from build123d import *

# Parameters (mm, degrees)
MOTOR_HOLDER_DEPTH = 15
SKETCH2_R          = 2.4
LEGO_MOUNT_DEPTH   = 7.76


with BuildPart() as part:
    # Sketch1 → Motor Holder (new body)
    with BuildSketch(Plane(origin=(0, 0, 0), x_dir=(0, 0, -1), z_dir=(1, 0, 0))):
        with BuildLine():
            Line((-8.959047103, 12.31), (8.959047103, 12.31))
            ThreePointArc((8.959047103, 12.31), (15.225, 0), (8.959047103, -12.31))
            Line((8.959047103, -12.31), (-8.959047103, -12.31))
            ThreePointArc((-8.959047103, -12.31), (-15.225, 0), (-8.959047103, 12.31))
        make_face()
        with BuildLine():
            Line((-7.923037612, 9.31), (7.923037612, 9.31))
            ThreePointArc((7.923037612, 9.31), (12.225, 0), (7.923037612, -9.31))
            Line((7.923037612, -9.31), (-7.923037612, -9.31))
            ThreePointArc((-7.923037612, -9.31), (-12.225, 0), (-7.923037612, 9.31))
        make_face(mode=Mode.SUBTRACT)
    extrude(amount=MOTOR_HOLDER_DEPTH)

    # Sketch2 → Lego Mount (add)
    # profile 1 of 2: a face of its own
    with BuildSketch(Plane.ZY):
        with BuildLine():
            Line((-7.97, 19.277326297), (7.97, 19.277326297))
            ThreePointArc((7.97, 19.277326297), (11.067073538, 16.640950889), (8.959047103, 13.162651831))
            Line((8.959047103, 13.162651831), (8.959047103, 12.31))
            Line((8.959047103, 12.31), (-8.959047103, 12.31))
            Line((-8.959047103, 12.31), (-8.959047103, 13.162651831))
            ThreePointArc((-8.959047103, 13.162651831), (-11.067073538, 16.640950889), (-7.97, 19.277326297))
        make_face()
        with Locations((-7.97, 16.14)):
            Circle(SKETCH2_R, mode=Mode.SUBTRACT)
        with Locations((0, 16.14)):
            Circle(SKETCH2_R, mode=Mode.SUBTRACT)
        with Locations((7.97, 16.14)):
            Circle(SKETCH2_R, mode=Mode.SUBTRACT)
    # profile 2 of 2: a face of its own
    with BuildSketch(Plane.ZY):
        with BuildLine():
            Line((-7.97, -19.277326297), (7.97, -19.277326297))
            ThreePointArc((7.97, -19.277326297), (11.067073538, -16.640950889), (8.959047103, -13.162651831))
            Line((8.959047103, -13.162651831), (8.959047103, -12.31))
            Line((8.959047103, -12.31), (-8.959047103, -12.31))
            Line((-8.959047103, -12.31), (-8.959047103, -13.162651831))
            ThreePointArc((-8.959047103, -13.162651831), (-11.067073538, -16.640950889), (-7.97, -19.277326297))
        make_face()
        with Locations(Location((7.97, -16.14, 0), (0, 0, 180))):
            Circle(SKETCH2_R, mode=Mode.SUBTRACT)
        with Locations(Location((0, -16.14, 0), (0, 0, 180))):
            Circle(SKETCH2_R, mode=Mode.SUBTRACT)
        with Locations(Location((-7.97, -16.14, 0), (0, 0, 180))):
            Circle(SKETCH2_R, mode=Mode.SUBTRACT)
    extrude(amount=-LEGO_MOUNT_DEPTH)


solid = part.part
Input: part model. Units: mm. Frame: model coordinates. A direction names the side the tool comes from. Give positions to 0.01 mm unless a question says otherwise; leave off trailing zeros. Order: outer loops, then holes, each group sorted by start corner. A loop starts at its lowest first (then second) coordinate and runs counter-clockwise, first axis right, second up. Notation, with made-up numbers: (-39.75, 36) - (-30.75, 36) arc R23 cw to (-30.75, 49) - close; hole circle Ø3 at (-30, 27.5). An arc over 180 degrees is marked (long way). Answer as a JSON object with one key per item and string values. Group by question number.
Q1. Line query: probe 1 along Z at (x, y) = (3.5, -16.14); probe 2 along Y at (x, z) = (6, 0); probe 3 along Y at (x, z) = (2.25, 6). Output: solid intervals per line, ascending.
Q2. Set-up query: faces 1 (the face through (4, -13, -8.959)), 2 (the face through (4, -13, 8.959)), 3 (the face through (7.395, 0.148, -12.224)), 4 (the face through (7.76, 16, 3)), 5 (the face through (7.76, -13, 0)). Return all of +Z, -Z, +X, -X, +Y, -Y with unobstructed straight access to the full face (end or side cutting, diameter ignored); none if empty.
Q3. Mould query, pull axis Z, two halves, no side actions, for faces 6 (the face through (7, 9.31, 0)), 7 (the face through (4, 13, -8.959)), 8 (the face through (4, -19.277, 0)). Classes: pulls with the +Z half, pulls with the -Z half, needs draft (parallel to the pull), parting line crosses it, or undercut.
Q4. Cut plane D-D, the plane x = 11.5. Output: boundary loops of the cut face in (y, z) (3 decimals), then the cut area to 3 significant figures.
Q5. Cut plane B-B, the plane x = 3.25. Output: boundary loops of the cut face in (y, z) (3 decimals).
Q6. Cut plane A-A, the plane z = 0. Output: boundary loops of the cut face in (x, y).
Q7. First-contact query: pin 1 Ø1.5 at (x, y) = (10, -4.5) entering from -Z; pin 2 Ø3 at (x, y) = (5.5, 8) entering from -Z; pin 3 Ø1 at (x, y) = (8, -9) entering from -Z. Flat tips, straight axial feed; report the tip coordinate or a pass-through.
Q8. Cut plane C-C, the plane y = 16.14. Output: boundary loops of the cut face in (x, z), then the cut area to 3 significant figures.
Results:
{
 "1": {"probe 1": "-11.11 to -10.37, -5.57 to -2.4, 2.4 to 5.57, 10.37 to 11.11", "probe 2": "-19.28 to -18.54, -13.74 to -9.31, 9.31 to 13.74, 18.54 to 19.28", "probe 3": "-19.28 to -17.51, -14.77 to -9.31, 9.31 to 14.77, 17.51 to 19.28"},
 "2": {"face 1": "-Z, +X, -X", "face 2": "+Z, +X, -X", "face 3": "+X, -X", "face 4": "+Z, -Z, +X, +Y", "face 5": "+Z, -Z, +X, -Y"},
 "3": {"face 6": "undercut", "face 7": "pulls with the -Z half", "face 8": "needs draft"},
 "4": {"outline": "(-12.31, -8.959) arc R15.225 ccw to (12.31, -8.959) - (12.31, 8.959) arc R15.225 ccw to (-12.31, 8.959) - close; hole (-9.31, -7.923) arc R12.225 ccw to (9.31, -7.923) - (9.31, 7.923) arc R12.225 ccw to (-9.31, 7.923) - close", "area": "251 mm^2"},
 "5": {"outline": "(-19.277, -7.97) arc R3.137 ccw to (-13.163, -8.959) - (-12.31, -8.959) arc R15.225 ccw to (12.31, -8.959) - (13.163, -8.959) arc R3.137 ccw to (19.277, -7.97) - (19.277, 7.97) arc R3.137 ccw to (13.163, 8.959) - (12.31, 8.959) arc R15.225 ccw to (-12.31, 8.959) - (-13.163, 8.959) arc R3.137 ccw to (-19.277, 7.97) - close; hole circle Ø4.8 at (-16.14, -7.97); hole circle Ø4.8 at (-16.14, 0); hole circle Ø4.8 at (-16.14, 7.97); hole (-9.31, -7.923) arc R12.225 ccw to (9.31, -7.923) - (9.31, 7.923) arc R12.225 ccw to (-9.31, 7.923) - close; hole circle Ø4.8 at (16.14, -7.97); hole circle Ø4.8 at (16.14, 0); hole circle Ø4.8 at (16.14, 7.97)"},
 "6": {"outline": "(0, -19.28) - (7.76, -19.28) - (7.76, -18.54) - (0, -18.54) - close; (0, -13.74) - (7.76, -13.74) - (7.76, -12.31) - (15, -12.31) - (15, -9.31) - (0, -9.31) - close; (0, 9.31) - (15, 9.31) - (15, 12.31) - (7.76, 12.31) - (7.76, 13.74) - (0, 13.74) - close; (0, 18.54) - (7.76, 18.54) - (7.76, 19.28) - (0, 19.28) - close"},
 "7": {"pin 1": "z = -14.76", "pin 2": "z = -13.77", "pin 3": "z = -12.63"},
 "8": {"outline": "(0, -11.11) - (7.76, -11.11) - (7.76, -10.37) - (0, -10.37) - close; (0, -5.57) - (7.76, -5.57) - (7.76, -2.4) - (0, -2.4) - close; (0, 2.4) - (7.76, 2.4) - (7.76, 5.57) - (0, 5.57) - close; (0, 10.37) - (7.76, 10.37) - (7.76, 11.11) - (0, 11.11) - close", "area": "60.6 mm^2"}
}
